Here's how the part is built. I have some questions about the finished solid (model axes, mm). Coordinates: 2 decimals unless noted, no trailing zeros. Loops run counter-clockwise (first coordinate to the right, second up) from the corner with the lowest first, then second, coordinate; pieces in that order, holes last. Notation, with made-up numbers: (57.5, 16.5) -> (111.5, 16.5) arc R28 ccw to (111.5, 40.5) -> close; hole circle Ø9 at (-2, -3). An arc over 180 degrees is marked (long way). Answer as a JSON object with one key per item and string values. Group by question number.
1) I want a section at B-B (z = 1.6). Write out the boundary of the cut face in (x, y), then the cut area to 3 significant figures.
2) I need wall thicknesses on probe 1 along X at (y, z) = (0, 2.9); probe 2 along Y at (x, z) = (1.5, 2). Which ranges of each line are inside material? Lowest first, please. Write a range as [from, to].
3) I want a section at D-D (y = -4.5). Write out the boundary of the cut face in (x, z).
4) If we mould it in two halves opening along X, with no side actions, what happens to faces 1 (the cylindrical face through (2.44, 0.54, 2.53)), 2 (the cylindrical face through (-4.715, 4.699, 2.535)), 3 (the flat face through (0, -5, 2)), 4 (the cylindrical face through (4.699, -4.715, 2.535))? For each: +X half, -X half, draft (parallel to the pull), parting line (faces both ways), or undercut.
5) I want a section at A-A (y = 0). Write out the boundary of the cut face in (x, z) (3 decimals).
```python
from build123d import *

# Parameters (mm, degrees)
SKETCH_1_W      = 10
SKETCH_1_H      = 10
EXTRUDE_1_DEPTH = 5
FILLET_1_R      = 1


with BuildPart() as part:
    # Эскиз1 → Бобышка-Вытянуть1 (new body)
    with BuildSketch(Plane.XY):
        Rectangle(SKETCH_1_W, SKETCH_1_H)
    extrude(amount=EXTRUDE_1_DEPTH)

    # Эскиз3 → Отверстие обработанное метчиком M61 (revolve, cut)
    with BuildSketch(Plane(origin=(0, 0, 5), x_dir=(0, -1, 0), z_dir=(1, 0, 0))):
        Polygon((0, 0), (0, 5), (3.025, 5), (2.5, 4.475), (2.5, 0.525), (3.025, 0), align=None)
    revolve(axis=Axis((0, 0, 11.35), (0, 0, -1)), mode=Mode.SUBTRACT)

    # Скругление1
    fillet_1_edges = [part.edges().sort_by_distance(p)[0] for p in [
        (5, -5, 2.5),
        (-5, -5, 2.5),
        (-5, 5, 2.5),
        (5, 5, 2.5),
    ]]
    fillet(fillet_1_edges, radius=FILLET_1_R)


solid = part.part
```
Determined:
{
 "1": {"outline": "(-5, -4) arc R1 ccw to (-4, -5) -> (4, -5) arc R1 ccw to (5, -4) -> (5, 4) arc R1 ccw to (4, 5) -> (-4, 5) arc R1 ccw to (-5, 4) -> close; hole circle Ø5 at (0, 0)", "area": "79.5 mm^2"},
 "2": {"probe 1": "[-5, -2.5], [2.5, 5]", "probe 2": "[-5, -2], [2, 5]"},
 "3": {"outline": "(-4.87, 0) -> (4.87, 0) -> (4.87, 5) -> (-4.87, 5) -> close"},
 "4": {"face 1": "undercut", "face 2": "-X half", "face 3": "draft", "face 4": "+X half"},
 "5": {"outline": "(-5, 0) -> (-3.025, 0) -> (-2.5, 0.525) -> (-2.5, 4.475) -> (-3.025, 5) -> (-5, 5) -> close; (2.5, 0.525) -> (3.025, 0) -> (5, 0) -> (5, 5) -> (3.025, 5) -> (2.5, 4.475) -> close"}
}
